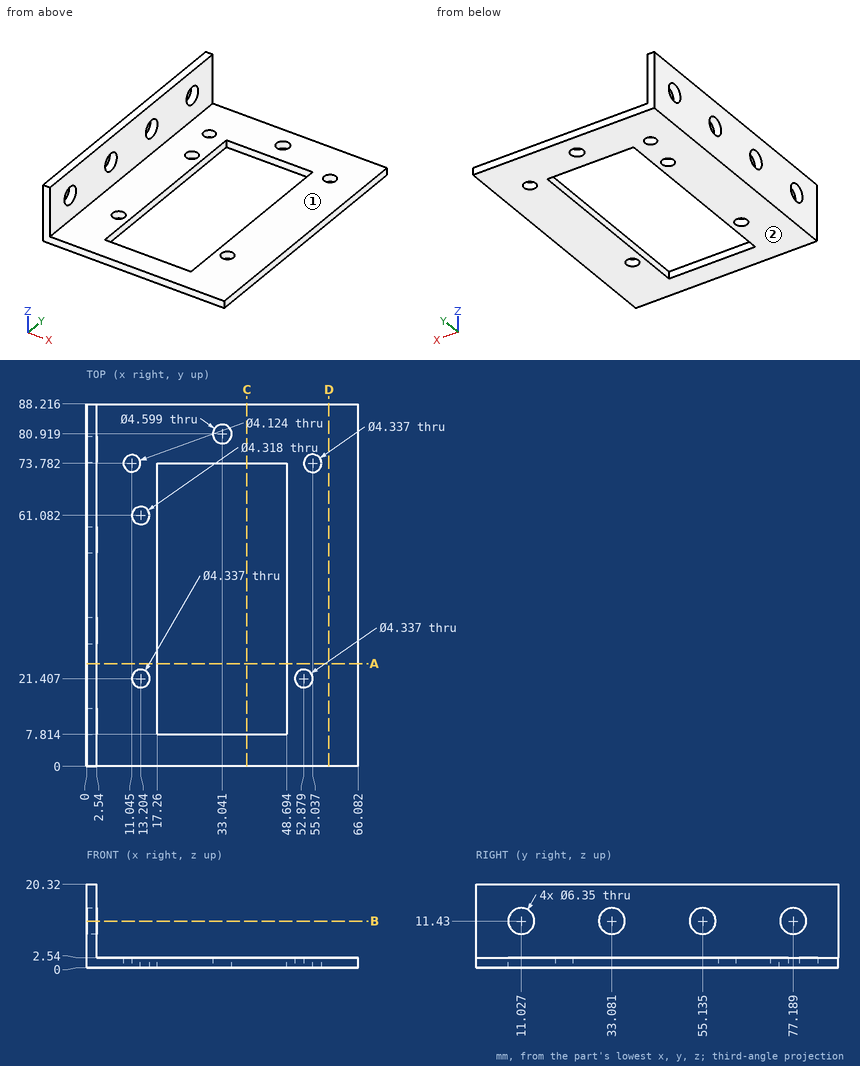
Source: three-view drawing plus pictorial views. Frame: mm from the lowest corner of the part. A direction names the side the tool comes from. Give positions to 0.01 mm unless a question says otherwise; leave off trailing zeros. Write each loop counter-clockwise with the first axis right and the second up, starting at its lowest first coordinate (ties: lowest second). Pieces come first, ordered by that corner, then holes. Notation, with made-up numbers: M 22,-12 L 77,-12 A19 cw 77,-3 Z; hole C 70,-15.75 d9. An arc over 180 degrees is marked long. Use one line per item in the form item = value.
1. Cut plane C-C on x = 39. Return loops of the section in (y, z) (1 decimal).
Outcome:
outline = M 0,0 L 7.8,0 L 7.8,2.5 L 0,2.5 Z; M 73.8,0 L 88.2,0 L 88.2,2.5 L 73.8,2.5 Z
2. First-contact query: P1, Ø4, axis at y = 25.5, z = 10.5, coming from the +X side; P2, Ø2, axis at x = 59, y = 32, coming from the +Z side; P3, Ø3.5, axis at x = 13.2, y = 61.08, coming from the +Z side. Flat tips, straight axial feed; report the tip coordinate or a pass-through.
Outcome:
P1 = 2.54
P2 = 2.54
P3 = through
3. Ray query, L1, parallel to Y at x = 13.5, z = 1.75 (1 decimal); L2, parallel to X at y = 44.5, z = 1.25; L3, parallel to Y at x = 39.5, z = 1 (1 decimal). Return the intervals inside material, ascending.
Outcome:
L1 = 0 to 19.3, 23.6 to 58.9, 63.2 to 88.2
L2 = 0 to 17.26, 48.69 to 66.08
L3 = 0 to 7.8, 73.8 to 88.2
4. Reachability of the marked faces 1 and 2 from +Z, -Z, +X, -X, +Y, -Y: full face, straight path, thin tool, end or side. Return the list, or none.
Outcome:
face_1 = +Z, +X, +Y, -Y
face_2 = -Z, +X, -X, +Y, -Y
5. Cut plane A-A on y = 25. Return loops of the section in (x, z), and give its area (3 significant figures).
Outcome:
outline = M 0,0 L 17.26,0 L 17.26,2.54 L 2.54,2.54 L 2.54,20.32 L 0,20.32 Z; M 48.69,0 L 66.08,0 L 66.08,2.54 L 48.69,2.54 Z
area = 133 mm²
6. Cut plane B-B on z = 11.43. Return loops of the section in (x, y) (1 decimal).
Outcome:
outline = M 0,0 L 2.5,0 L 2.5,7.9 L 0,7.9 Z; M 0,14.2 L 2.5,14.2 L 2.5,29.9 L 0,29.9 Z; M 0,36.3 L 2.5,36.3 L 2.5,52 L 0,52 Z; M 0,58.3 L 2.5,58.3 L 2.5,74 L 0,74 Z; M 0,80.4 L 2.5,80.4 L 2.5,88.2 L 0,88.2 Z
7. Cut plane D-D on x = 59. Return loops of the section in (y, z) (1 decimal), and give its area (3 significant figures).
Outcome:
outline = M 0,0 L 88.2,0 L 88.2,2.5 L 0,2.5 Z
area = 224 mm²
